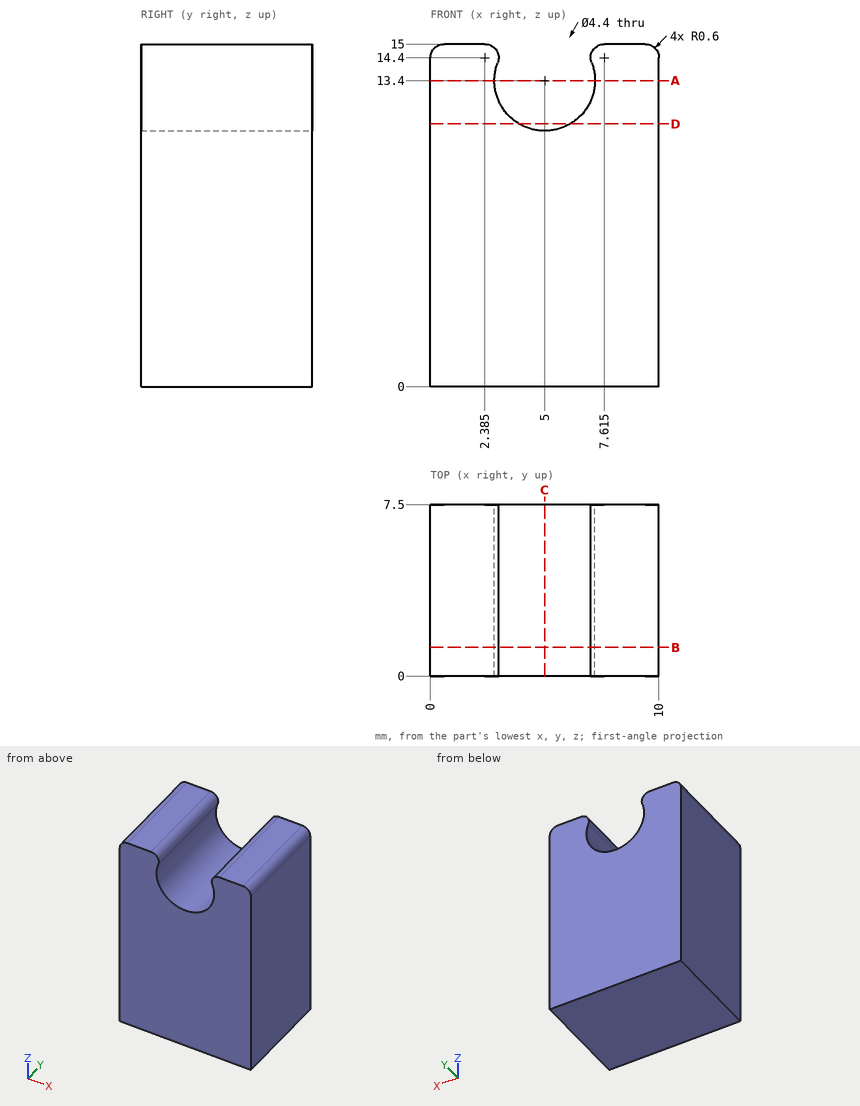
Geometry: see drawing. Coordinates: mm, zero at the bounding-box minimum. Round coordinates to 2 decimals unless told otherwise and drop trailing zeros. Write each loop counter-clockwise with the first axis right and the second up, starting at its lowest first coordinate (ties: lowest second). Pieces come first, ordered by that corner, then holes. Notation, with made-up numbers: M -20.5,32.25 L 19.5,32.25 A24 cw 19.5,59.25 Z; hole C 6,37 d1. An arc over 180 degrees is marked long. Answer as a JSON object with one key per item and string values. Group by question number.
(1) Section query D-D on z = 11.5. Output: boundary loops of the cut face in (x, y).
(2) Section query A-A on z = 13.4. Output: boundary loops of the cut face in (x, y), then the cut area to 3 significant figures.
(3) Section query B-B on y = 1.25. Output: boundary loops of the cut face in (x, z) (1 decimal).
(4) Section query C-C on x = 5. Output: boundary loops of the cut face in (y, z), then the cut area to 3 significant figures.
(5) Ray query, line 1 (X direction, y = 5, z = 13.4); line 2 (X direction, y = 6.5, z = 11.5); line 3 (Z direction, x = 4.5, y = 6). Return the intervals inside material, ascending. Write a range as [from, to].
Computed values:
{
 "1": {"outline": "M 0,0 L 3.89,0 L 3.89,7.5 L 0,7.5 Z; M 6.11,0 L 10,0 L 10,7.5 L 6.11,7.5 Z"},
 "2": {"outline": "M 0,0 L 2.8,0 L 2.8,7.5 L 0,7.5 Z; M 7.2,0 L 10,0 L 10,7.5 L 7.2,7.5 Z", "area": "42.0 mm^2"},
 "3": {"outline": "M 0,0 L 10,0 L 10,14.4 A0.6 ccw 9.4,15 L 7.6,15 A0.6 ccw 7.1,14.2 A2.2 cw long 2.9,14.2 A0.6 ccw 2.4,15 L 0.6,15 A0.6 ccw 0,14.4 Z"},
 "4": {"outline": "M 0,0 L 7.5,0 L 7.5,11.2 L 0,11.2 Z", "area": "84.0 mm^2"},
 "5": {"line 1": "[0, 2.8], [7.2, 10]", "line 2": "[0, 3.89], [6.11, 10]", "line 3": "[0, 11.26]"}
}
